from build123d import *

# Parameters (mm, degrees)
SKETCH4_W           = 6
SKETCH4_H           = 40
SKETCH4_W_2         = 8
BOSS_EXTRUDE4_DEPTH = 5
SKETCH6_W           = 6
SKETCH6_H           = 40
SKETCH6_W_2         = 8
BOSS_EXTRUDE5_DEPTH = 15
SKETCH7_R           = 3
CUT_EXTRUDE2_DEPTH  = 73.773621595
CUT_EXTRUDE3_REACH  = 74.774
CUT_EXTRUDE4_REACH  = 90.566
CUT_EXTRUDE5_REACH  = 92.449
SKETCH10_R          = 2.1
CHAMFER1_SIZE       = 2
FILLET1_R           = 4.8
SKETCH11_R          = 2
BOSS_EXTRUDE6_DEPTH = 4
BOSS_EXTRUDE7_DEPTH = 4


with BuildPart() as part:
    # Sketch4 → Boss-Extrude4 (new body)
    with BuildSketch(Plane(origin=(0, 0, 0), x_dir=(1, 0, 0), z_dir=(0, 1, 0))):
        Polygon((0, 60), (0, 0), (66, 0), (66, 60), (56, 60), (56, 50), (62, 50), (62, 10), (56, 10), (56, 20), (50, 20), (42, 20), (36, 20), (30, 20), (30, 60), align=None)
        with Locations((39, 40)):
            Rectangle(SKETCH4_W, SKETCH4_H)
        with Locations((33, 40)):
            Rectangle(SKETCH4_W, SKETCH4_H)
        with Locations((46, 40)):
            Rectangle(SKETCH4_W_2, SKETCH4_H)
        Polygon((56, 50), (56, 60), (50, 60), (50, 20), (56, 20), align=None)
        Polygon((62, 50), (56, 50), (56, 20), (56, 10), (62, 10), align=None)
    extrude(amount=BOSS_EXTRUDE4_DEPTH)

    # Sketch6 → Boss-Extrude5 (add)
    with BuildSketch(Plane(origin=(0, 5, 0), x_dir=(1, 0, 0), z_dir=(0, 1, 0))):
        with Locations((33, 40)):
            Rectangle(SKETCH6_W, SKETCH6_H)
        with Locations((46, 40)):
            Rectangle(SKETCH6_W_2, SKETCH6_H)
        Polygon((62, 50), (56, 50), (56, 20), (56, 10), (62, 10), align=None)
    boss_extrude5 = extrude(amount=BOSS_EXTRUDE5_DEPTH)

    # Sketch7 → Cut-Extrude2 (cut, through all)
    with BuildSketch(Plane.ZY.offset(-30)):
        with Locations(Location((-40, 13, 0), (0, 0, 180))):
            Circle(SKETCH7_R)
    cut_extrude2 = extrude(amount=-CUT_EXTRUDE2_DEPTH, mode=Mode.SUBTRACT)

    # Cut-Extrude3: up to this face of the body (flat: up to its plane)
    cut_extrude3_end = Plane(part.part.faces().sort_by_distance((50, 12.5, -20.427200187))[0])
    # Sketch8 → Cut-Extrude3 (cut, up to the picked face)
    with BuildSketch(Plane.ZY.offset(-30), mode=Mode.PRIVATE) as cut_extrude3_sk1:
        with BuildLine():
            Line((-60, 20), (-60, 5))
            Line((-60, 5), (-44.570704164, 18.30176041))
            ThreePointArc((-44.570704164, 18.30176041), (-42.437998885, 19.561719396), (-40, 20))
            Line((-40, 20), (-60, 20))
        make_face()
    cut_extrude3_tool1 = split(extrude(cut_extrude3_sk1.sketch, amount=-CUT_EXTRUDE3_REACH, mode=Mode.PRIVATE), bisect_by=cut_extrude3_end, keep=Keep.BOTH, mode=Mode.PRIVATE)
    # Sketch8 → Cut-Extrude3 (cut, up to the picked face)
    with BuildSketch(Plane.ZY.offset(-30), mode=Mode.PRIVATE) as cut_extrude3_sk2:
        with BuildLine():
            Line((-35.429295836, 18.30176041), (-20, 5))
            Line((-20, 5), (-20, 20))
            Line((-20, 20), (-40, 20))
            ThreePointArc((-40, 20), (-37.562001115, 19.561719396), (-35.429295836, 18.30176041))
        make_face()
    cut_extrude3_tool2 = split(extrude(cut_extrude3_sk2.sketch, amount=-CUT_EXTRUDE3_REACH, mode=Mode.PRIVATE), bisect_by=cut_extrude3_end, keep=Keep.BOTH, mode=Mode.PRIVATE)
    cut_extrude3_1 = cut_extrude3_tool1.solids().sort_by(Axis((30, 15.027454, -54.131076), (1, 0, 0)))[0]
    add(cut_extrude3_1, mode=Mode.SUBTRACT)
    cut_extrude3_2 = cut_extrude3_tool2.solids().sort_by(Axis((30, 15.027454, -25.868924), (1, 0, 0)))[0]
    add(cut_extrude3_2, mode=Mode.SUBTRACT)
    cut_extrude3 = cut_extrude3_1 + cut_extrude3_2  # Cut-Extrude3 as one shape, for the pattern or mirror that repeats it

    # Sketch9 → Cut-Extrude4 (cut, up to next)
    with BuildSketch(Plane(origin=(62, 0, 0), x_dir=(0, 0, -1), z_dir=(1, 0, 0)), mode=Mode.PRIVATE) as cut_extrude4_sk1:
        with BuildLine():
            ThreePointArc((36.717902336, 19.182866239), (38.30885596, 19.792645422), (40, 20))
            Line((40, 20), (10, 20))
            Line((10, 20), (10, 5))
            Line((10, 5), (36.717902336, 19.182866239))
        make_face()
    cut_extrude4_tool1 = extrude(cut_extrude4_sk1.sketch, amount=-CUT_EXTRUDE4_REACH, mode=Mode.PRIVATE) & part.part
    # Sketch9 → Cut-Extrude4 (cut, up to next)
    with BuildSketch(Plane(origin=(62, 0, 0), x_dir=(0, 0, -1), z_dir=(1, 0, 0)), mode=Mode.PRIVATE) as cut_extrude4_sk2:
        with BuildLine():
            ThreePointArc((40, 20), (44.104331221, 18.67049074), (46.649592052, 15.186990065))
            Line((46.649592052, 15.186990065), (50, 5))
            Line((50, 5), (50, 20))
            Line((50, 20), (40, 20))
        make_face()
    cut_extrude4_tool2 = extrude(cut_extrude4_sk2.sketch, amount=-CUT_EXTRUDE4_REACH, mode=Mode.PRIVATE) & part.part
    cut_extrude4_1 = cut_extrude4_tool1.solids().sort_by_distance((62, 15.005539, -19.440707))[0]
    add(cut_extrude4_1, mode=Mode.SUBTRACT)
    cut_extrude4_2 = cut_extrude4_tool2.solids().sort_by_distance((62, 15.452907, -47.894979))[0]
    add(cut_extrude4_2, mode=Mode.SUBTRACT)
    cut_extrude4 = cut_extrude4_1 + cut_extrude4_2  # Cut-Extrude4 as one shape, for the pattern or mirror that repeats it

    # Mirror1: Boss-Extrude5, Cut-Extrude2, Cut-Extrude3, Cut-Extrude4 across plane
    add(boss_extrude5.mirror(Plane.ZY.offset(-33)))
    add(cut_extrude2.mirror(Plane.ZY.offset(-33)), mode=Mode.SUBTRACT)
    add(cut_extrude3.mirror(Plane.ZY.offset(-33)), mode=Mode.SUBTRACT)
    add(cut_extrude4.mirror(Plane.ZY.offset(-33)), mode=Mode.SUBTRACT)

    # Sketch10 → Cut-Extrude5 (cut, up to next)
    with BuildSketch(Plane(origin=(0, 5, 0), x_dir=(1, 0, 0), z_dir=(0, 1, 0)), mode=Mode.PRIVATE) as cut_extrude5_sk1:
        with Locations(Location((5.1, 54.9, 0), (0, 0, 270))):
            Circle(SKETCH10_R)
    cut_extrude5_tool1 = extrude(cut_extrude5_sk1.sketch, amount=-CUT_EXTRUDE5_REACH, mode=Mode.PRIVATE) & part.part
    # Sketch10 → Cut-Extrude5 (cut, up to next)
    with BuildSketch(Plane(origin=(0, 5, 0), x_dir=(1, 0, 0), z_dir=(0, 1, 0)), mode=Mode.PRIVATE) as cut_extrude5_sk2:
        with Locations(Location((60.9, 54.9, 0), (0, 0, 270))):
            Circle(SKETCH10_R)
    cut_extrude5_tool2 = extrude(cut_extrude5_sk2.sketch, amount=-CUT_EXTRUDE5_REACH, mode=Mode.PRIVATE) & part.part
    # Sketch10 → Cut-Extrude5 (cut, up to next)
    with BuildSketch(Plane(origin=(0, 5, 0), x_dir=(1, 0, 0), z_dir=(0, 1, 0)), mode=Mode.PRIVATE) as cut_extrude5_sk3:
        with Locations(Location((60.9, 5.1, 0), (0, 0, 270))):
            Circle(SKETCH10_R)
    cut_extrude5_tool3 = extrude(cut_extrude5_sk3.sketch, amount=-CUT_EXTRUDE5_REACH, mode=Mode.PRIVATE) & part.part
    # Sketch10 → Cut-Extrude5 (cut, up to next)
    with BuildSketch(Plane(origin=(0, 5, 0), x_dir=(1, 0, 0), z_dir=(0, 1, 0)), mode=Mode.PRIVATE) as cut_extrude5_sk4:
        with Locations(Location((5.1, 5.1, 0), (0, 0, 270))):
            Circle(SKETCH10_R)
    cut_extrude5_tool4 = extrude(cut_extrude5_sk4.sketch, amount=-CUT_EXTRUDE5_REACH, mode=Mode.PRIVATE) & part.part
    add(cut_extrude5_tool1.solids().sort_by_distance((5.1, 5, -54.9))[0], mode=Mode.SUBTRACT)
    add(cut_extrude5_tool2.solids().sort_by_distance((60.9, 5, -54.9))[0], mode=Mode.SUBTRACT)
    add(cut_extrude5_tool3.solids().sort_by_distance((60.9, 5, -5.1))[0], mode=Mode.SUBTRACT)
    add(cut_extrude5_tool4.solids().sort_by_distance((5.1, 5, -5.1))[0], mode=Mode.SUBTRACT)

    # Chamfer1
    chamfer1_edges = [part.edges().sort_by_distance(p)[0] for p in [
        (5.1, 5, -7.2),
        (60.9, 5, -7.2),
        (60.9, 5, -57),
        (5.1, 5, -57),
    ]]
    chamfer(chamfer1_edges, length=CHAMFER1_SIZE)

    # Fillet1
    fillet1_edges = [part.edges().sort_by_distance(p)[0] for p in [
        (66, 2.5, 0),
        (0, 2.5, 0),
        (0, 2.5, -60),
        (66, 2.5, -60),
    ]]
    fillet(fillet1_edges, radius=FILLET1_R)

    # Sketch11 → Boss-Extrude6 (add)
    with BuildSketch(Plane(origin=(0, 5, 0), x_dir=(1, 0, 0), z_dir=(0, 1, 0))):
        with Locations(Location((19, 11, 0), (0, 0, 270))):
            Circle(SKETCH11_R)
        with Locations(Location((47, 11, 0), (0, 0, 270))):
            Circle(SKETCH11_R)
    extrude(amount=BOSS_EXTRUDE6_DEPTH)

    # Sketch12 → Boss-Extrude7 (add)
    with BuildSketch(Plane.ZY.offset(-4)):
        Polygon((-45.1, 10.055513627), (-45.1, 15.944486373), (-46.1, 15.944486373), (-46.1, 5), (-33.9, 5), (-33.9, 15.944486373), (-34.9, 15.944486373), (-34.9, 10.055513627), (-40, 7.111027254), align=None)
    extrude(amount=BOSS_EXTRUDE7_DEPTH)


solid = part.part
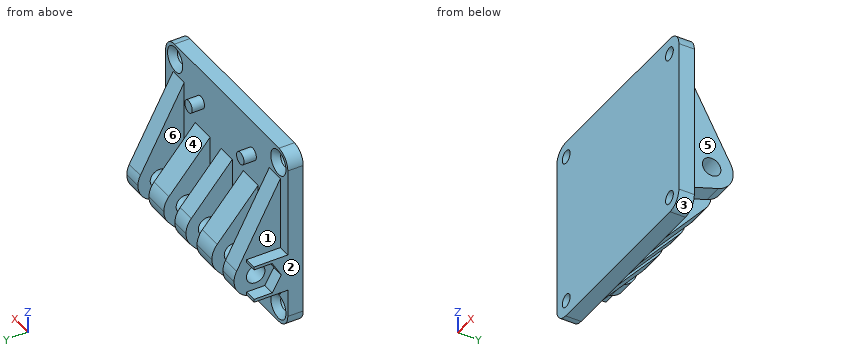
The listing builds one solid part. Answer for the finished solid, in the listing's coordinates (mm). Face numbers are marked on the shaded views. A direction names the side the tool comes from. Coordinates: 2 decimals unless noted, no trailing zeros. Loops run counter-clockwise (first coordinate to the right, second up) from the corner with the lowest first, then second, coordinate; pieces in that order, holes last.
1) A tool of negligible diameter and unlimited length cuts with its end or side. For the marked faces 4, 5 and 6, from which of +Z, -Z, +X, -X, +Y, -Y can it reach the whole face along a straight path? Write none if from no direction.
2) Find section C-C on y = 17.5. Write down the section's boundary in (x, z).
3) Find section B-B on x = 19. Write down the section's boundary in (y, z).
4) Find section A-A on y = 8.25. Give the number of separate pieces and of enclosed holes in the cut face, then the cut area to 3 significant figures.
5) Flat-ended cylindrical pins translate along their axes: pin 1 Ø5 at (x, z) = (37.5, -27) entering from +Y; pin 2 Ø5 at (x, z) = (5.1, -54.9) entering from +Y; pin 3 Ø2 at (x, y) = (1.5, 13) entering from +Z; pin 4 Ø1 at (y, z) = (12, -20) entering from -X. Find the tip coordinate at first contact, or state that the pin passes through.
6) Find the intervals of material crossed by L1, parallel to X at y = 1.2, z = -5.1; L2, parallel to X at y = 5.75, z = -30; L3, parallel to X at y = 8.5, z = -37.5, in increasing order.
7) Find section D-D on z = -11. Write down the section's boundary in (x, y).
8) Determine the mould class of the marked faces 1, 2 and 3 for opening direction Z: pulls with the +Z half, pulls with the -Z half, needs draft (parallel to the pull), parting line crosses it, or undercut.
Values:
1. face 4: +Y
1. face 5: +Z, -Z, +X, +Y
1. face 6: +Z, -Z, +Y
2. outline: (4, -45.36) - (10, -45.36) - (10, -33.55) - (4, -33.55) - close; (16, -45.5) - (24, -45.5) - (24, -34.5) - (16, -34.5) - close; (30, -45.5) - (36, -45.5) - (36, -34.5) - (30, -34.5) - close; (42, -45.5) - (50, -45.5) - (50, -34.5) - (42, -34.5) - close; (56, -45.36) - (62, -45.36) - (62, -33.55) - (56, -33.55) - close
3. outline: (0, -60) - (5, -60) - (18.3, -44.57) arc R7 ccw to (18.3, -35.43) - (5, -20) - (5, -13) - (9, -13) - (9, -9) - (5, -9) - (5, 0) - (0, 0) - close; hole circle Ø6 at (13, -40)
4. separate pieces: 7
4. enclosed holes: 0
4. area: 1,170 mm2
5. pin 1: stops at y = 12.76
5. pin 2: stops at y = 3.4
5. pin 3: stops at z = -33.9
5. pin 4: passes through
6. L1: x = 0 to 3, 7.2 to 58.8, 63 to 66
6. L2: x = 4 to 10, 16 to 24, 30 to 36, 42 to 50, 56 to 62
6. L3: x = 0 to 10, 16 to 24, 30 to 36, 42 to 50, 56 to 62
7. outline: (0, 0) - (66, 0) - (66, 5) - (62, 5) - (62, 5.53) - (56, 5.53) - (56, 5) - (49, 5) - (49, 9) - (45, 9) - (45, 5) - (21, 5) - (21, 9) - (17, 9) - (17, 5) - (10, 5) - (10, 5.53) - (4, 5.53) - (4, 5) - (0, 5) - close
8. face 1: undercut
8. face 2: needs draft
8. face 3: pulls with the -Z half
